Autodesk Fusion 360 part; units mm, degrees
sketch "Sketch1" plane through (0, 0, 0) normal (0, 0, 1) x (1, 0, 0)
  line L0 (0, 0) -> (70, 0)
  line L1 (70, 0) -> (70, 65)
  line L2 (70, 65) -> (0, 65)
  line L3 (0, 65) -> (0, 0)
  dimension "d1" = 70
  dimension "d2" = 65
extrude "Extrude1" add sketch "Sketch1" along normal blind 2.5
sketch "Sketch2" plane through (0, 0, 2.5) normal (0, 0, 1) x (-1, 0, 0)
  line L0 (0, -65) -> (0, 0)
  line L1 (0, 0) -> (-70, 0)
  line L2 (-70, 0) -> (-70, -65)
  line L3 (-70, -65) -> (0, -65)
  line L4 (0, -65) -> (-2, -65)
  line L5 (-2, -65) -> (-2, 0)
  line L6 (-2, 0) -> (0, 0)
  line L7 (0, 0) -> (0, -65)
  line L8 (-70, -65) -> (-68, -65)
  line L9 (-68, -65) -> (-68, 0)
  line L10 (-68, 0) -> (-70, 0)
  line L11 (-70, 0) -> (-70, -65)
  line L12 (0, -65) -> (-70, -65)
  line L13 (-70, -65) -> (-70, -63)
  line L14 (-70, -63) -> (0, -63)
  line L15 (0, -63) -> (0, -65)
  line L16 (0, 0) -> (-70, 0)
  line L17 (-70, 0) -> (-70, -2)
  line L18 (-70, -2) -> (0, -2)
  line L19 (0, -2) -> (0, 0)
  dimension "d5" = 2
  dimension "d6" = 2
  dimension "d7" = 65
  dimension "d8" = 2
  dimension "d9" = 2
extrude "Extrude2" add sketch "Sketch2" along normal blind 30 contours L0 L3 L4 L5 L7 L12 L14 L15 | L0 L5 L7 L14 L18 | L3 L5 L9 L12 L14 | L0 L1 L5 L6 L7 L16 L18 L19 | L2 L3 L8 L9 L11 L12 L13 L14 | L1 L5 L9 L16 L18 | L2 L9 L11 L14 L18 | L1 L2 L9 L10 L11 L16 L17 L18
sketch "Sketch3" plane through (0, 0, 2.5) normal (0, 0, 1) x (-1, 0, 0)
  line L0 (-2, -2) -> (-68, -2)
  line L1 (-68, -2) -> (-68, -63)
  line L2 (-68, -63) -> (-2, -63)
  line L3 (-2, -63) -> (-2, -2)
  circle A0 centre (-6.2, -6.3) radius 1.5
  circle A1 centre (-6.2, -58.8) radius 1.5
  circle A2 centre (-64.77, -58.8) radius 1.5
  circle A3 centre (-64.77, -6.3) radius 1.5
  dimension "d12" = 3
  dimension "d13" = 3
  dimension "d14" = 3
  dimension "d15" = 3
  dimension "d16" = 58.57
  dimension "d17" = 58.57
  dimension "d18" = 52.5
  dimension "d19" = 52.5
extrude "Extrude3" cut sketch "Sketch3" against normal blind 2.5 contours A0 | A1 | A2 | A3
sketch "Sketch6" plane through (0, 0, 0) normal (0, -1, 0) x (1, 0, 0)
  line L0 (0, 0) -> (70, 0)
  line L1 (70, 0) -> (70, 32.5)
  line L2 (70, 32.5) -> (0, 32.5)
  line L3 (0, 32.5) -> (0, 0)
  line L4 (14.5, 2.5) -> (26.5, 2.5)
  line L5 (26.5, 2.5) -> (26.5, 10.5)
  line L6 (26.5, 10.5) -> (14.5, 10.5)
  line L7 (14.5, 10.5) -> (14.5, 2.5)
  line L8 (11.75, 18.25) -> (58.25, 18.25)
  arc A0 (58.25, 18.25) -> (58.25, 21.75) centre (58.25, 20) ccw
  line L9 (58.25, 21.75) -> (11.75, 21.75)
  arc A1 (11.75, 21.75) -> (11.75, 18.25) centre (11.75, 20) ccw
  line L10 (10, 20) -> (60, 20) construction
  dimension "d32" = 12
  dimension "d33" = 8
  dimension "d34" = 2.5
  dimension "d35" = 14.5
  dimension "d36" = 3.5
sketch "Sketch7" plane through (0, 0, 0) normal (-1, 0, 0) x (0, -1, 0)
  line L0 (-65, 0) -> (0, 0)
  line L1 (0, 0) -> (0, 32.5)
  line L2 (0, 32.5) -> (-65, 32.5)
  line L3 (-65, 32.5) -> (-65, 0)
  line L4 (-48.5, 6.2) -> (-21.5, 6.2)
  line L5 (-21.5, 6.2) -> (-21.5, 32.5)
  line L6 (-21.5, 32.5) -> (-48.5, 32.5)
  line L7 (-48.5, 32.5) -> (-48.5, 6.2)
  dimension "d37" = 16.5
  dimension "d38" = 6.2
  dimension "d47" = 27
  dimension "d48" = 26.3
extrude "Extrude6" cut sketch "Sketch7" against normal blind 2 contours L2 L4 L5 L6 L7
extrude "Extrude7" cut sketch "Sketch6" against normal blind 2 contours L4 L5 L6 L7 | L8 A0 L9 A1
sketch "Sketch8" plane through (0, 65, 0) normal (0, 1, 0) x (-1, 0, 0)
  line L0 (-70, 0) -> (0, 0)
  line L1 (0, 0) -> (0, 32.5)
  line L2 (0, 32.5) -> (-70, 32.5)
  line L3 (-70, 32.5) -> (-70, 0)
  line L4 (-58.25, 23.25) -> (-11.75, 23.25)
  arc A0 (-11.75, 23.25) -> (-11.75, 26.75) centre (-11.75, 25) ccw
  line L5 (-11.75, 26.75) -> (-58.25, 26.75)
  arc A1 (-58.25, 26.75) -> (-58.25, 23.25) centre (-58.25, 25) ccw
  line L6 (-60, 25) -> (-10, 25) construction
  line L7 (-58.25, 8.25) -> (-11.75, 8.25)
  arc A2 (-11.75, 8.25) -> (-11.75, 11.75) centre (-11.75, 10) ccw
  line L8 (-11.75, 11.75) -> (-58.25, 11.75)
  arc A3 (-58.25, 11.75) -> (-58.25, 8.25) centre (-58.25, 10) ccw
  line L9 (-60, 10) -> (-10, 10) construction
  dimension "d43" = 3.5
  dimension "d44" = 3.5
extrude "Extrude8" cut sketch "Sketch8" against normal blind 2 contours L4 A0 L5 A1 | L7 A2 L8 A3
fillet "Fillet1" radius 1 4 edges at (70, 0, 16.25) (0, 0, 16.25) (70, 65, 16.25) (0, 65, 16.25)
Geometry check sheet. Reference: the model listing, model coordinates, mm. A direction names the side the tool comes from. Coordinates: 2 decimals unless noted, no trailing zeros. Order: outer loops, then holes, each group sorted by start corner. A loop starts at its lowest first (then second) coordinate and runs counter-clockwise, first axis right, second up. Notation, with made-up numbers: (-4, 12.25) - (6, 12.25) arc R21 ccw to (6, 17.25) - close; hole circle Ø6 at (3, 50). An arc over 180 degrees is marked (long way). One line per item, written item: value.
(1) Depth check by flat-ended pin: pin 1 Ø1.8 at (x, y) = (64.77, 6.3) entering from +Z; pin 2 Ø1.5 at (y, z) = (39.5, 12) entering from -X; pin 3 Ø1.6 at (x, y) = (1, 39.5) entering from +Z; pin 4 Ø6 at (x, y) = (14, 21.5) entering from +Z. Enter the tip coordinate at first touch or a pass-through.
Data:
pin 1: passes through
pin 2: stops at x = 68
pin 3: stops at z = 6.2
pin 4: stops at z = 2.5
(2) Thickness scan on probe 1 along Y at (x, z) = (6.2, 0.95); probe 2 along X at (y, z) = (6.3, 1.8); probe 3 along X at (y, z) = (9, 21). Record the ranges inside material, lowest first. Write a range as from..to.
Data:
probe 1: y = 0..4.8, 7.8..57.3, 60.3..65
probe 2: x = 0..4.7, 7.7..63.27, 66.27..70
probe 3: x = 0..2, 68..70
(3) Sectioned sample at C-C (x = 55.5). Enter the section's corners in (y, z), and give its area (4 significant figures).
Data:
outline: (0, 0) - (65, 0) - (65, 8.25) - (63, 8.25) - (63, 2.5) - (2, 2.5) - (2, 18.25) - (0, 18.25) - close; (0, 21.75) - (2, 21.75) - (2, 32.5) - (0, 32.5) - close; (63, 11.75) - (65, 11.75) - (65, 23.25) - (63, 23.25) - close; (63, 26.75) - (65, 26.75) - (65, 32.5) - (63, 32.5) - close
area: 261.5 mm^2
(4) Access from +Z, -Z, +X, -X, +Y, -Y to the whole of each face (thin tool, end or side, straight path). Record for faces 5 (the face through (35, 64, 8.25)), 6 (the face through (68, 33, 17)), 7 (the face through (1, 21.5, 19)), 8 (the face through (35, 1, 18.25)), 9 (the face through (21, 1, 10.5)).
Data:
face 5: +Y
face 6: +Z
face 7: +Z, -X
face 8: -Y
face 9: +Y, -Y
(5) Sectioned sample at A-A (x = 23). Enter the section's corners in (y, z).
Data:
outline: (0, 0) - (65, 0) - (65, 8.25) - (63, 8.25) - (63, 2.5) - (0, 2.5) - close; (0, 10.5) - (2, 10.5) - (2, 18.25) - (0, 18.25) - close; (0, 21.75) - (2, 21.75) - (2, 32.5) - (0, 32.5) - close; (63, 11.75) - (65, 11.75) - (65, 23.25) - (63, 23.25) - close; (63, 26.75) - (65, 26.75) - (65, 32.5) - (63, 32.5) - close
(6) Sectioned sample at D-D (z = 14.5). Enter the section's corners in (x, y).
Data:
outline: (0, 1) arc R1 ccw to (1, 0) - (69, 0) arc R1 ccw to (70, 1) - (70, 64) arc R1 ccw to (69, 65) - (1, 65) arc R1 ccw to (0, 64) - (0, 48.5) - (2, 48.5) - (2, 63) - (68, 63) - (68, 2) - (2, 2) - (2, 21.5) - (0, 21.5) - close
(7) Sectioned sample at B-B (z = 20). Enter the section's corners in (x, y).
Data:
outline: (0, 1) arc R1 ccw to (1, 0) - (10, 0) - (10, 2) - (2, 2) - (2, 21.5) - (0, 21.5) - close; (0, 48.5) - (2, 48.5) - (2, 63) - (68, 63) - (68, 2) - (60, 2) - (60, 0) - (69, 0) arc R1 ccw to (70, 1) - (70, 64) arc R1 ccw to (69, 65) - (1, 65) arc R1 ccw to (0, 64) - close
(8) Release check for a two-part mould opening along Z. For faces 1 (the face through (26.5, 1, 6)), 2 (the face through (0, 33, 5)), 3 (the face through (69, 32, 32.5)), 4 (the face through (35, 64, 23.25)) record: +Z half, -Z half, draft (parallel to the pull), parting line (faces both ways), or undercut.
Data:
face 1: undercut
face 2: draft
face 3: +Z half
face 4: undercut
